Source: CAD feature listing. Evaluate the final solid. Frame: model axes, mm. Face numbers are marked on the shaded views. A direction names the side the tool comes from. Give positions to 0.01 mm unless a question says otherwise; leave off trailing zeros. Order: outer loops, then holes, each group sorted by start corner. A loop starts at its lowest first (then second) coordinate and runs counter-clockwise, first axis right, second up.
1) Section D-D, the plane z = 0.5. Return loops of the section in (x, y) (1 decimal).
2) Section A-A, the plane y = 0. Give the number of separate pieces and of enclosed holes in the cut face, plus the area to 3 significant figures.
3) Material intervals for line 1 (X direction, y = 0.25, z = 3); line 2 (Y direction, x = 0, z = 5.5) (3 decimals); line 3 (Z direction, x = 9, y = -7) (3 decimals), sorted ascending.
4) Draft query along Y for the marked faces 1, 2 and 3. Return one class per face: released by +Y, released by -Y, zero draft, split by the parting line, or undercut.
5) Section B-B, the plane z = 4. Return loops of the section in (x, y) (3 decimals).
6) Access query for the marked faces 4 and 5. Directions: +Z, -Z, +X, -X, +Y, -Y. A direction counts if a zero-diameter tool reaches every point of the face in a straight line with its end or side. Return the directions, or none.
7) First-contact query: P1, Ø2, axis at y = -11, z = 3, coming from the +X side; P2, Ø4, axis at x = 7, y = 4.5, coming from the +Z side (3 decimals); P3, Ø1, axis at y = 11.5, z = 1, coming from the +X side. Flat tips, straight axial feed; report the tip coordinate or a pass-through.
```python
from build123d import *

# Parameters (mm, degrees)
F0_R     = 14.605
F0_R_2   = 12.065
F1_DEPTH = 9.525
F0_R_3   = 1.5
F2_DEPTH = 3.175
F4_R     = 18.379294
F4_R_2   = 13.335
F5_DEPTH = 1.5875


with BuildPart() as f1:
    # F0 (on Top) → F1 (new body)
    with BuildSketch(Plane.XY):
        Circle(F0_R)
        Circle(F0_R_2, mode=Mode.SUBTRACT)
    extrude(amount=F1_DEPTH)

    # F0 (on Top) → F2 (join)
    with BuildSketch(Plane.XY):
        Circle(F0_R_2)
        with Locations((-4.7625, 0)):
            Circle(F0_R_3, mode=Mode.SUBTRACT)
        with Locations((4.7625, 0)):
            Circle(F0_R_3, mode=Mode.SUBTRACT)
    extrude(amount=F2_DEPTH)

    # F4 (on offset) → F5 (cut)
    with BuildSketch(Plane.XY.offset(6.35)):
        Circle(F4_R)
        Circle(F4_R_2, mode=Mode.SUBTRACT)
    extrude(amount=-F5_DEPTH, mode=Mode.SUBTRACT)


solid = f1.part
```
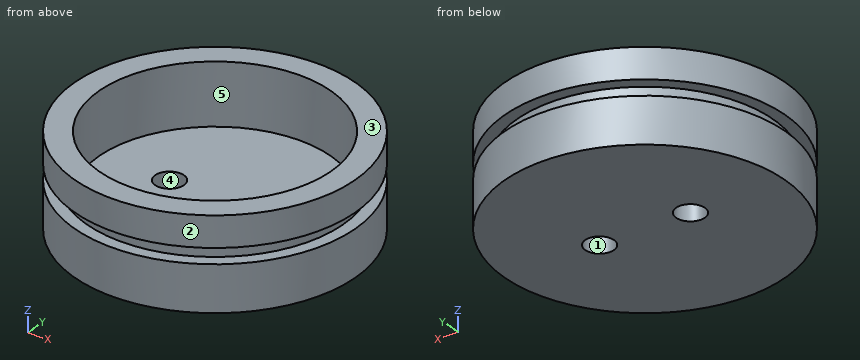
From the geometry:
1. outline: circle Ø29.2 at (0, 0); hole circle Ø3 at (-4.8, 0); hole circle Ø3 at (4.8, 0)
2. separate pieces: 3
2. enclosed holes: 0
2. area: 102 mm2
3. line 1: x = -14.6 to -6.24, -3.28 to 3.28, 6.24 to 14.6
3. line 2: y = -13.335 to -12.065, 12.065 to 13.335
3. line 3: z = 0 to 3.175
4. face 1: undercut
4. face 2: split by the parting line
4. face 3: zero draft
5. outline: circle Ø29.21 at (0, 0); hole circle Ø24.13 at (0, 0)
6. face 4: +Z, -Z
6. face 5: +Z
7. P1: stops at x = 10.64
7. P2: stops at z = 3.175
7. P3: stops at x = 9.61
